from build123d import *

# Parameters (mm, degrees)
SALIENTE_EXTRUIR1_DEPTH = 3
CROQUIS2_W              = 170
CROQUIS2_H              = 48.2
SALIENTE_EXTRUIR2_DEPTH = 3


with BuildPart() as part:
    # Croquis1 → Saliente-Extruir1 (new body)
    with BuildSketch(Plane.XY):
        with BuildLine():
            Line((-98.745, 15), (-91.041526265, 15))
            ThreePointArc((-91.041526265, 15), (-88.803264961, 14.746290901), (-86.678577108, 13.998037267))
            Line((-86.678577108, 13.998037267), (-8.316422892, -23.998037267))
            ThreePointArc((-8.316422892, -23.998037267), (-6.191735039, -24.746290901), (-3.953473735, -25))
            Line((-3.953473735, -25), (78.589355629, -25))
            ThreePointArc((78.589355629, -25), (83.859818396, -26.501634144), (87.547419794, -30.555555556))
            ThreePointArc((87.547419794, -30.555555556), (107.583834765, -33.838834765), (104.300555556, -13.802419794))
            ThreePointArc((104.300555556, -13.802419794), (100.246634144, -10.114818396), (98.745, -4.844355629))
            Line((98.745, -4.844355629), (98.745, 15))
            ThreePointArc((98.745, 15), (95.816067812, 22.071067812), (88.745, 25))
            Line((88.745, 25), (-81.424491924, 25))
            ThreePointArc((-81.424491924, 25), (-86.424491924, 26.339745962), (-90.084745962, 30))
            ThreePointArc((-90.084745962, 30), (-107.405254038, 30), (-98.745, 15))
        make_face()
    extrude(amount=SALIENTE_EXTRUIR1_DEPTH)


with BuildPart() as body_2:
    # Simetría2: mirrored copy
    add(part.part.mirror(Plane.XY.offset(-21.1)))


with BuildPart() as part_1:
    add(part.part)

    add(body_2.part)  # Saliente-Extruir2 merges body 2
    # Croquis2 → Saliente-Extruir2 (add)
    with BuildSketch(Plane(origin=(0, 25, 0), x_dir=(1, 0, 0), z_dir=(0, 1, 0))):
        with Locations((3.745, 21.1)):
            Rectangle(CROQUIS2_W, CROQUIS2_H)
    extrude(amount=-SALIENTE_EXTRUIR2_DEPTH)


solid = part_1.part
Read the model definition and answer for the solid it produces. Units are mm, in the model's axes. A direction names the side the tool comes from. Round coordinates to 2 decimals unless told otherwise and drop trailing zeros. Write each loop counter-clockwise with the first axis right and the second up, starting at its lowest first coordinate (ties: lowest second). Pieces come first, ordered by that corner, then holes.
1. Determine the mould class of faces 1 (the face through (24, -1, 0)), 2 (the face through (24, -1, -45.2)), 3 (the face through (100.3, -10.2, -43.7)) for opening direction Z: pulls with the +Z half, pulls with the -Z half, needs draft (parallel to the pull), parting line crosses it, or undercut.
2. Which of the six approach directions +Z, -Z, +X, -X, +Y, -Y give full straight-line access (tool end or side, diameter ignored) to faces 4 (the face through (3, 22, -21)), 5 (the face through (95.893, 21.993, -43.679))?
3. Given pin 1 Ø0.9 at (x, z) = (-95.5, 1.5) entering from -Y; pin 2 Ø1.5 at (x, z) = (-73, -2) entering from +Y; pin 3 Ø0.9 at (y, z) = (8, -44) entering from +X (3 decimals), each flat-ended and moving along its own axis, determine where each tip first touches the part or whether it passes through.
4. The part is cut by section A-A, the plane x = 20. Determine the outline of the cut face in (y, z), then the cut area to 3 significant figures.
5. The part is cut by section B-B, the plane y = 2. Determine the outline of the cut face in (x, z) (3 decimals), then the cut area to 3 significant figures.
6. Straight lines are drawn through the part: L1, parallel to Z at x = -72, y = 13.5; L2, parallel to Y at x = -49, z = -30; L3, parallel to Y at x = -42.5, z = -42.5. For each, find the intervals that lie inside material, in ascending order.
7. The part is cut by section C-C, the plane z = -12. Determine the outline of the cut face in (x, y) (3 decimals), then the cut area to 3 significant figures.
Values:
1. face 1: undercut
1. face 2: pulls with the -Z half
1. face 3: needs draft
2. face 4: +X, -X, -Y
2. face 5: +Z, -Z, +X, +Y
3. pin 1: stops at y = 15
3. pin 2: stops at y = 25
3. pin 3: stops at x = 98.745
4. outline: (-25, -45.2) - (25, -45.2) - (25, 3) - (-25, 3) - (-25, 0) - (22, 0) - (22, -42.2) - (-25, -42.2) - close
4. area: 427 mm2
5. outline: (-61.934, -45.2) - (98.745, -45.2) - (98.745, -42.2) - (-61.934, -42.2) - close; (-61.934, 0) - (98.745, 0) - (98.745, 3) - (-61.934, 3) - close
5. area: 964 mm2
6. L1: z = -45.2 to -42.2, 0 to 3
6. L2: y = 22 to 25
6. L3: y = -7.42 to 25
7. outline: (-81.255, 22) - (88.745, 22) - (88.745, 25) - (-81.255, 25) - close
7. area: 510 mm2
